The model under review builds one solid part; all positions refer to its coordinate system, in mm. Face numbers are marked on the shaded views. Round coordinates to 2 decimals unless told otherwise and drop trailing zeros. Order: outer loops, then holes, each group sorted by start corner. A loop starts at its lowest first (then second) coordinate and runs counter-clockwise, first axis right, second up. Notation, with made-up numbers: (56, 63) -> (67, 63) arc R12 cw to (67, 86) -> close; hole circle Ø5 at (34.25, 59). An arc over 180 degrees is marked (long way). Return JSON: item names as keys, results as strings. Group by question number.
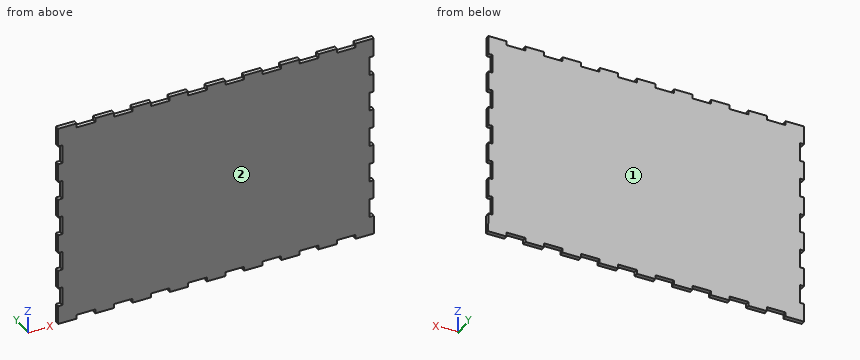
from build123d import *

# Parameters (mm, degrees)
F1_DEPTH = 3


with BuildPart() as f1:
    # F0 (on Front) → F1 (new body)
    with BuildSketch(Plane.XZ):
        Polygon((113.2355, 61.363636), (113.2355, 75), (100.097, 75), (100.097, 71.999997), (86.7637, 71.999997), (86.7637, 75), (73.4307, 75), (73.4307, 72), (60.0974, 72), (60.0974, 75), (46.7641, 75), (46.7641, 72), (33.4308, 72), (33.4308, 75), (20.0975, 75), (20.0975, 72), (6.7642, 72), (6.7642, 75), (-6.5691, 75), (-6.5691, 72), (-19.9024, 72), (-19.9024, 75), (-33.2357, 75), (-33.2357, 72), (-46.569, 72), (-46.569, 75), (-59.9023, 75), (-59.9023, 72), (-73.2356, 72), (-73.2356, 75), (-86.5689, 75), (-86.5689, 72), (-99.9022, 72), (-99.9022, 75), (-113.2355, 75), (-113.2355, 61.363636), (-110.2355, 61.363636), (-110.2355, 47.727273), (-113.2355, 47.727273), (-113.2355, 34.090909), (-110.2355, 34.090909), (-110.2355, 20.454545), (-113.2355, 20.454545), (-113.2355, 6.818182), (-110.2355, 6.818182), (-110.2355, -6.818182), (-113.2355, -6.818182), (-113.2355, -20.454545), (-110.2355, -20.454545), (-110.2355, -34.090909), (-113.2355, -34.090909), (-113.2355, -47.727273), (-110.2355, -47.727273), (-110.2355, -61.363636), (-113.2355, -61.363636), (-113.2355, -75), (-99.9022, -75), (-99.9022, -72), (-86.5689, -72), (-86.5689, -75), (-73.2356, -75), (-73.2356, -72), (-59.9023, -72), (-59.9023, -75), (-46.569, -75), (-46.569, -72), (-33.2357, -72), (-33.2357, -75), (-19.9024, -75), (-19.9024, -72), (-6.5691, -72), (-6.5691, -75), (6.7642, -75), (6.7642, -72), (20.0975, -72), (20.0975, -75), (33.4308, -75), (33.4308, -72), (46.7641, -72), (46.7641, -75), (60.0974, -75), (60.0974, -72), (73.4307, -72), (73.4307, -75), (86.7637, -75), (86.7637, -71.999997), (100.097, -71.999997), (100.097, -75), (113.2355, -75), (113.4308, -75), (113.2355, -61.363636), (110.2355, -61.363636), (110.2355, -47.727273), (113.2355, -47.727273), (113.2355, -34.090909), (110.2355, -34.090909), (110.2355, -20.454545), (113.2355, -20.454545), (113.2355, -6.818182), (110.2355, -6.818182), (110.2355, 6.818182), (113.2355, 6.818182), (113.2355, 20.454545), (110.2355, 20.454545), (110.2355, 34.090909), (113.2355, 34.090909), (113.2355, 47.727273), (110.2355, 47.727273), (110.2355, 61.363636), align=None)
    extrude(amount=F1_DEPTH)


solid = f1.part
Item 1: Consider section B-B on x = 36. State the section outline as (y, z) points.
Item 2: The part is to be moulded in two halves that separate along Y. For the marked faces 1 and 2, say which applies: +Y half, -Y half, draft (parallel to the pull), parting line (faces both ways), or undercut.
Item 3: Consider section A-A on z = -2. State the section outline as (x, y) points.
Item 4: Insertion check: pin 1 Ø1.5 at (y, z) = (-1.5, 42) entering from +X; pin 2 Ø1 at (x, y) = (-39, -2) entering from +Z; pin 3 Ø0.9 at (y, z) = (-1.5, -73) entering from +X. Each pin has a flat end and moves straight along its axis. Give the tip position at first contact, or say it passes through.
Item 5: Wall thickness on line 1 along X through (y, z) = (-1.7, -52.5); line 2 along Z through (x, y) = (44, -2.15); line 3 along X through (y, z) = (-2.3, 16.5): over which ranges is each line inside the solid? List them lowest first.
Values:
{
 "1": {"outline": "(-3, -72) -> (0, -72) -> (0, 72) -> (-3, 72) -> close"},
 "2": {"face 1": "+Y half", "face 2": "-Y half"},
 "3": {"outline": "(-110.24, -3) -> (110.24, -3) -> (110.24, 0) -> (-110.24, 0) -> close"},
 "4": {"pin 1": "x = 113.24", "pin 2": "z = 72", "pin 3": "x = 113.41"},
 "5": {"line 1": "-110.24 to 110.24", "line 2": "-72 to 72", "line 3": "-113.24 to 113.24"}
}
